Can you work these out from the model? Positions are in its coordinate system, mm. A direction names the side the tool comes from. Give positions to 0.01 mm unless a question says otherwise; leave off trailing zeros. Write each loop counter-clockwise with the first axis right and the second up, starting at its lowest first coordinate (ties: lowest second). Pieces come first, ordered by that corner, then holes.
```python
from build123d import *

# Parameters (mm, degrees)
EXTRUDE_2_DEPTH     = 85
EXTRUDE_3_DEPTH     = 20
SKETCH_5_W          = 40
SKETCH_5_H          = 20
EXTRUDE_4_DEPTH     = 40
FILLET_1_R          = 20
SKETCH_6_R          = 10
CUT_EXTRUDE_1_DEPTH = 20


with BuildPart() as part:
    # 스케치1 → 보스-돌출2 (new body)
    with BuildSketch(Plane.XY):
        with BuildLine():
            Line((-24, -15.199619772), (-65, -15.199619772))
            Line((-65, -15.199619772), (-65, -0.199619772))
            Line((-65, -0.199619772), (-29, -0.199619772))
            Line((-29, -0.199619772), (-29, 20.142585551))
            Line((-29, 20.142585551), (29, 20.142585551))
            Line((29, 20.142585551), (29, -0.199619772))
            Line((29, -0.199619772), (65, -0.199619772))
            Line((65, -0.199619772), (65, -15.199619772))
            Line((65, -15.199619772), (24, -15.199619772))
            ThreePointArc((24, -15.199619772), (0, 8.800380228), (-24, -15.199619772))
        make_face()
    extrude(amount=EXTRUDE_2_DEPTH)

    # 스케치4 → 보스-돌출3 (add)
    with BuildSketch(Plane(origin=(0, 0, 0), x_dir=(-1, 0, 0), z_dir=(0, 0, -1))):
        Polygon((-65, -0.199619772), (-29, -0.199619772), (-29, 20.142585551), (29, 20.142585551), (29, -0.199619772), (65, -0.199619772), (20.923247903, 60.800380228), (-19.076752097, 60.800380228), align=None)
    extrude(amount=-EXTRUDE_3_DEPTH)

    # 스케치5 → 보스-돌출4 (add)
    with BuildSketch(Plane.XY.offset(20)):
        with Locations((-0.923247903, 50.800380228)):
            Rectangle(SKETCH_5_W, SKETCH_5_H)
    extrude(amount=EXTRUDE_4_DEPTH)

    # 필렛1
    fillet_1_edges = [part.edges().sort_by_distance(p)[0] for p in [
        (-20.923247903, 50.800380228, 60),
        (19.076752097, 50.800380228, 60),
    ]]
    fillet(fillet_1_edges, radius=FILLET_1_R - 0.0001)  # a hair under: the kernel refuses the full size

    # 스케치6 → 컷-돌출1 (cut)
    with BuildSketch(Plane(origin=(0, 60.800380228, 0), x_dir=(1, 0, 0), z_dir=(0, 1, 0))):
        with Locations(Location((-0.923247903, -40, 0), (0, 0, 180))):
            Circle(SKETCH_6_R)
    extrude(amount=-CUT_EXTRUDE_1_DEPTH, mode=Mode.SUBTRACT)


solid = part.part
```
1) Suppose I cut it at C-C on x = 47.5. Write out the boundary of the cut face in (y, z).
Values follow:
outline: (-15.2, 0) - (23.05, 0) - (23.05, 20) - (-0.2, 20) - (-0.2, 85) - (-15.2, 85) - close
2) For pin 1 Ø2 at (y, z) = (0, 32.5) entering from -X; pin 2 Ø3 at (y, z) = (19.5, 26.5) entering from +X; pin 3 Ø10 at (y, z) = (20, 10) entering from +X; pin 4 Ø12 at (x, z) = (-7.5, 65.5) entering from -Y, each with a flat end and sliding along its axis, tell me the tip position at first contact or that it passes through.
Values follow:
pin 1: stops at x = -65
pin 2: stops at x = 29
pin 3: stops at x = 53.56
pin 4: stops at y = 4.64
3) Suppose I cut it at D-D on z = 33.5. Write out the boundary of the cut face in (x, y), plus the area to 3 significant figures.
Values follow:
outline: (-65, -15.2) - (-24, -15.2) arc R24 cw to (24, -15.2) - (65, -15.2) - (65, -0.2) - (29, -0.2) - (29, 20.14) - (-29, 20.14) - (-29, -0.2) - (-65, -0.2) - close; (-20.92, 40.8) - (-8.52, 40.8) - (-8.52, 60.8) - (-20.92, 60.8) - close; (6.68, 40.8) - (19.08, 40.8) - (19.08, 60.8) - (6.68, 60.8) - close
area: 2,720 mm2
4) For faces 4 (the face through (-6, 40.8, 31)), 5 (the face through (19.077, 51, 30)), 6 (the face through (-15.22, 50.94, 53.986)), which set-ups out of +Z, -Z, +X, -X, +Y, -Y let a thin tool reach every point of the face, with its end or its side?
Values follow:
face 4: +Z, +X, -X
face 5: +Z, +X, +Y
face 6: +Z, -X, +Y
5) If we mould it in two halves opening along Y, with no side actions, what happens to faces 1 (the face through (41.717, 30.727, 9.86)), 2 (the face through (-29, 10, 52)), 3 (the face through (1, 24, 20))? For each: +Y half, -Y half, draft (parallel to the pull), parting line (faces both ways), or undercut.
Values follow:
face 1: +Y half
face 2: draft
face 3: undercut
6) Please list where these lines run through material, in increasing order: L1, parallel to Y at x = -0.5, z = 56.5; L2, parallel to Y at x = 34, z = 59.5; L3, parallel to Z at x = 22, y = 30.
Values follow:
L1: y = 8.8 to 20.14, 40.8 to 60.8
L2: y = -15.2 to -0.2
L3: z = 0 to 20
7) Suppose I cut it at A-A on z = 46.5. Write out the boundary of the cut face in (x, y).
Values follow:
outline: (-65, -15.2) - (-24, -15.2) arc R24 cw to (24, -15.2) - (65, -15.2) - (65, -0.2) - (29, -0.2) - (29, 20.14) - (-29, 20.14) - (-29, -0.2) - (-65, -0.2) - close; (-19.84, 40.8) - (-8.52, 40.8) - (-8.52, 60.8) - (-19.84, 60.8) - close; (6.68, 40.8) - (17.99, 40.8) - (17.99, 60.8) - (6.68, 60.8) - close
